```python
from build123d import *

# Parameters (mm, degrees)
SKETCH1_W           = 58.42
SKETCH1_H           = 58.42
BOSS_EXTRUDE1_DEPTH = 50.8
SKETCH2_R           = 6
BOSS_EXTRUDE2_DEPTH = 76.2


with BuildPart() as part:
    # Sketch1 → Boss-Extrude1 (new body)
    with BuildSketch(Plane(origin=(0, 0, 0), x_dir=(1, 0, 0), z_dir=(0, 1, 0))):
        with Locations((0, -3.030175439)):
            Rectangle(SKETCH1_W, SKETCH1_H)
    extrude(amount=BOSS_EXTRUDE1_DEPTH)

    # Sketch2 → Boss-Extrude2 (add)
    with BuildSketch(Plane(origin=(0, 50.8, 0), x_dir=(1, 0, 0), z_dir=(0, 1, 0))):
        Circle(SKETCH2_R)
    extrude(amount=BOSS_EXTRUDE2_DEPTH)


solid = part.part
```
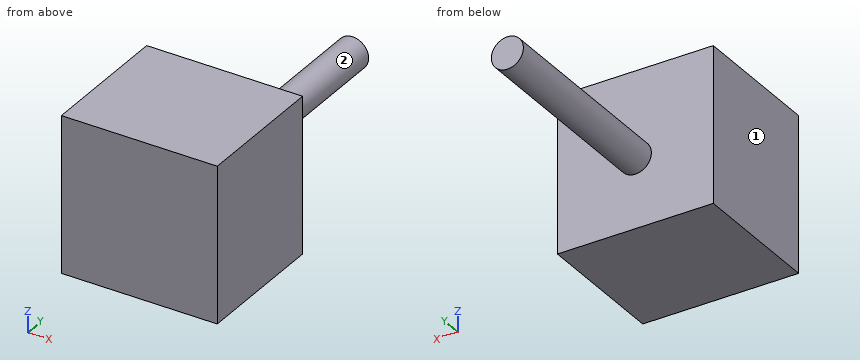
Geometry check sheet. Reference: the model listing, model coordinates, mm. Face numbers are marked on the shaded views. A direction names the side the tool comes from. Give positions to 0.01 mm unless a question says otherwise; leave off trailing zeros. Write each loop counter-clockwise with the first axis right and the second up, starting at its lowest first coordinate (ties: lowest second). Pieces come first, ordered by that corner, then holes.
1) Gauge pin test, flat ends, axial feed: pin 1 (10 mm diameter, centred on x = 2.5, z = 14.5, fed in from +Y); pin 2 (4 mm diameter, centred on x = 8, z = -13, fed in from -Y). Record the tip position at first contact, or that the pin passes through.
2) Section check D-D, the plane z = 23. Record the boundary of the cut face in (x, y), and give its area (3 significant figures).
3) Section check B-B, the plane z = 0. Record the boundary of the cut face in (x, y).
4) Section check C-C, the plane y = 104.5. Record the boundary of the cut face in (x, z).
5) Material ranges on L1, parallel to Y at x = -11, z = 17; L2, parallel to X at y = 59.5, z = 0.5, recorded low to high.
6) Section check A-A, the plane x = 0. Record the boundary of the cut face in (y, z), and give its area (3 significant figures).
7) Access from +Z, -Z, +X, -X, +Y, -Y to the whole of each face (thin tool, end or side, straight path). Record for the marked faces 1 and 2.
Computed:
1. pin 1: stops at y = 50.8
1. pin 2: stops at y = 0
2. outline: (-29.21, 0) - (29.21, 0) - (29.21, 50.8) - (-29.21, 50.8) - close
2. area: 2,970 mm2
3. outline: (-29.21, 0) - (29.21, 0) - (29.21, 50.8) - (6, 50.8) - (6, 127) - (-6, 127) - (-6, 50.8) - (-29.21, 50.8) - close
4. outline: circle Ø12 at (0, 0)
5. L1: y = 0 to 50.8
5. L2: x = -5.98 to 5.98
6. outline: (0, -26.18) - (50.8, -26.18) - (50.8, -6) - (127, -6) - (127, 6) - (50.8, 6) - (50.8, 32.24) - (0, 32.24) - close
6. area: 3,880 mm2
7. face 1: +Z, -Z, -X, +Y, -Y
7. face 2: +Y
